Geometry check sheet. Reference: the model listing, model coordinates, mm. A direction names the side the tool comes from. Round coordinates to 2 decimals unless told otherwise and drop trailing zeros. Order: outer loops, then holes, each group sorted by start corner. A loop starts at its lowest first (then second) coordinate and runs counter-clockwise, first axis right, second up. Notation, with made-up numbers: (88, 77.5) - (137, 77.5) arc R26 ccw to (137, 106.5) - close; hole circle Ø7 at (63, 76). An arc over 180 degrees is marked (long way). One line per question, with ' | ' between items. Start each with the question number.
Q1. Material ranges on line 1 along X through (y, z) = (36.5, 225.5); line 2 along Y through (x, z) = (876.5, 688); line 3 along Z through (x, y) = (544.5, 543.5), recorded low to high.
Q2. Sectioned sample at A-A, the plane x = 41.5. Enter the section's corners in (y, z).
Q3. Sectioned sample at D-D, the plane x = 615. Enter the section's corners in (y, z), then the cut area to 3 significant figures.
Q4. Tool access check on faces 5 (the face through (905, 67.986, 394)), 6 (the face through (453, -32.014, 801)), 7 (the face through (55.569, 537, 394)). Record the directions out of +Z, -Z, +X, -X, +Y, -Y that give a thin tool (end or side, any length) a straight path to the whole face; none if there is none.
Q5. Gauge pin test, flat end, axial feed: P1, Ø3, axis at x = 353, y = 300, coming from the -Z side. Record the tip position at first contact, or that the pin passes through.
Q6. Mould release check, pull along X, two halves, no side actions. Record for faces 1 (the face through (-44.431, 506, 517)), 2 (the face through (955.569, 506, 517)), 3 (the face through (5, 539, 0)), 4 (the face through (55.569, 17, 394)): +X half, -X half, draft (parallel to the pull), parting line (faces both ways), or undercut.
Q7. Sectioned sample at C-C, the plane y = 513. Enter the section's corners in (x, z).
Q8. Sectioned sample at B-B, the plane z = 236. Enter the section's corners in (x, y), then the cut area to 3 significant figures.
```python
from build123d import *

# Parameters (mm, degrees)
F0_W     = 1000
F0_H     = 620
F1_DEPTH = 850
F2_W     = 1000
F2_H     = 420
F3_DEPTH = 800
F4_W     = 800
F4_H     = 620
F5_DEPTH = 800


with BuildPart() as f1:
    # F0 (on Top) → F1 (new body)
    with BuildSketch(Plane.XY):
        with Locations((455.56918, 277.985783)):
            Rectangle(F0_W, F0_H)
    extrude(amount=F1_DEPTH)

    # F2 (on Top) → F3 (cut)
    with BuildSketch(Plane.XY):
        with Locations((455.56918, 277.985783)):
            Rectangle(F2_W, F2_H)
    extrude(amount=F3_DEPTH, mode=Mode.SUBTRACT)

    # F4 (on Top) → F5 (cut)
    with BuildSketch(Plane.XY):
        with Locations((455.56918, 277.985783)):
            Rectangle(F4_W, F4_H)
    extrude(amount=F5_DEPTH, mode=Mode.SUBTRACT)


solid = f1.part
```
Determined:
1) line 1: x = -44.43 to 55.57, 855.57 to 955.57 | line 2: y = -32.01 to 67.99, 487.99 to 587.99 | line 3: z = 800 to 850
2) outline: (-32.01, 0) - (67.99, 0) - (67.99, 800) - (487.99, 800) - (487.99, 0) - (587.99, 0) - (587.99, 850) - (-32.01, 850) - close
3) outline: (-32.01, 800) - (587.99, 800) - (587.99, 850) - (-32.01, 850) - close | area: 31,000 mm2
4) face 5: -Z, +X, -X | face 6: +Z, -Z, +X, -X, -Y | face 7: -Z, +Y, -Y
5) P1: stops at z = 800
6) face 1: -X half | face 2: +X half | face 3: draft | face 4: undercut
7) outline: (-44.43, 0) - (55.57, 0) - (55.57, 800) - (855.57, 800) - (855.57, 0) - (955.57, 0) - (955.57, 850) - (-44.43, 850) - close
8) outline: (-44.43, -32.01) - (55.57, -32.01) - (55.57, 67.99) - (-44.43, 67.99) - close; (-44.43, 487.99) - (55.57, 487.99) - (55.57, 587.99) - (-44.43, 587.99) - close; (855.57, -32.01) - (955.57, -32.01) - (955.57, 67.99) - (855.57, 67.99) - close; (855.57, 487.99) - (955.57, 487.99) - (955.57, 587.99) - (855.57, 587.99) - close | area: 40,000 mm2
